```python
from build123d import *

# Parameters (mm, degrees)
SKETCH_R        = 22.5
SKETCH_R_2      = 19
PAD_DEPTH       = 10
CHAMFER_SIZE    = 1
CHAMFER001_SIZE = 1


with BuildPart() as part:
    # Sketch → Pad (new body)
    with BuildSketch(Plane.XY):
        Circle(SKETCH_R)
        Circle(SKETCH_R_2, mode=Mode.SUBTRACT)
    extrude(amount=PAD_DEPTH)

    # Chamfer
    chamfer_edges = [part.edges().sort_by_distance(p)[0] for p in [
        (-19, 0, 10),
    ]]
    chamfer(chamfer_edges, length=CHAMFER_SIZE)

    # Chamfer001
    chamfer001_edges = [part.edges().sort_by_distance(p)[0] for p in [
        (-22.5, 0, 0),
    ]]
    chamfer(chamfer001_edges, length=CHAMFER001_SIZE)


solid = part.part
```
Build history of the part. All positions in model axes, mm. Round coordinates to 2 decimals unless told otherwise and drop trailing zeros. Order: outer loops, then holes, each group sorted by start corner. A loop starts at its lowest first (then second) coordinate and runs counter-clockwise, first axis right, second up. Notation, with made-up numbers: (-24, -25.75) -> (31, -25.75) arc R32 ccw to (31, 7.25) -> close; hole circle Ø5 at (26.25, 68.25). An arc over 180 degrees is marked (long way). Answer in a Markdown table with one row per item.
1) Band-saw the part on B-B on z = 7.5. Give the cut face in (x, y).
Values:
| item | result |
|---|---|
| outline | circle Ø45 at (0, 0); hole circle Ø38 at (0, 0) |
2) Pin check, flat tips, straight feed: P1, Ø1.5, axis at y = -16, z = 4, coming from the +X side; P2, Ø3, axis at x = -7, z = 3.5, coming from the -Y side; P3, Ø3, axis at x = 16.5, y = 14, coming from the -Z side; P4, Ø4, axis at x = 0.5, z = 3, coming from the -Y side. Stop position of each tip, or through.
Values:
| item | result |
|---|---|
| P1 | x = 16.54 |
| P2 | y = -21.82 |
| P3 | z = 0 |
| P4 | y = -22.5 |
3) Mould opens along Y. For faces 1 (the cylindrical face through (10.382, -19.961, 5.437)), 2 (the flat face through (-20.1, -1.6, 10)), 3 (the cylindrical face through (8.767, -16.856, 4.437)) say: released by +Y, released by -Y, zero draft, split by the parting line, or undercut.
Values:
| item | result |
|---|---|
| face 1 | split by the parting line |
| face 2 | zero draft |
| face 3 | undercut |
4) Band-saw the part on A-A on x = 0. Give the cut face in (y, z), and give its area (3 significant figures).
Values:
| item | result |
|---|---|
| outline | (-22.5, 1) -> (-21.5, 0) -> (-19, 0) -> (-19, 9) -> (-20, 10) -> (-22.5, 10) -> close; (19, 0) -> (21.5, 0) -> (22.5, 1) -> (22.5, 10) -> (20, 10) -> (19, 9) -> close |
| area | 68.0 mm2 |
5) Wall check: L1, parallel to Y at x = 0.5, z = 8; L2, parallel to X at y = 8, z = 6.75; L3, parallel to Y at x = 7, z = 2.5. Give the ranges that are in metal, low to high.
Values:
| item | result |
|---|---|
| L1 | -22.49 to -18.99, 18.99 to 22.49 |
| L2 | -21.03 to -17.23, 17.23 to 21.03 |
| L3 | -21.38 to -17.66, 17.66 to 21.38 |
